Geometry: final body of the model. Coordinates: model frame, mm. Coordinates: 2 decimals unless noted, no trailing zeros. Loops run counter-clockwise (first coordinate to the right, second up) from the corner with the lowest first, then second, coordinate; pieces in that order, holes last. Notation, with made-up numbers: (32.25, -4) - (60.25, -4) arc R33 ccw to (60.25, 29) - close; hole circle Ø9 at (36, -10). An arc over 180 degrees is marked (long way). Put each result on its own line as item: value. Start each with the question number.
1) Section B-B on x = -31.55. Output: boundary loops of the cut face in (y, z), and give its area (3 significant figures).
2) Draft query along Y for faces 1 (the cylindrical face through (23.78, -24.3, 0.99)), 2 (the cylindrical face through (-0.1, 29.05, 0.99)), 3 (the cylindrical face through (24.3, 23.78, 0.99)). Return one class per face: +Y half, -Y half, draft (parallel to the pull), parting line (faces both ways), or undercut.
3) Material intervals for line 1 along Y through (x, z) = (0, 1.4); line 2 along X through (y, z) = (-1.5, 1.65); line 3 along Y through (x, z) = (-2, 0.7), sorted ascending. Write a range as from..to.
4) Section C-C on z = 1.6. Output: boundary loops of the cut face in (x, y).
5) Section A-A on y = 7.5. Output: boundary loops of the cut face in (x, z), and give its area (3 significant figures).
6) Section D-D on x = 24. Output: boundary loops of the cut face in (y, z).
7) Contact query for flat-ended pins moving along their axis: pin 1 Ø1 at (y, z) = (8, 1) entering from -X; pin 2 Ø5 at (x, y) = (-10, 11.5) entering from +Z. Output: stop coordinate, or through.
```python
from build123d import *

# Parameters (mm, degrees)
CYLINDER_R     = 2.5
CYLINDER_DEPTH = 10
ARRAY_COUNT    = 4
TUBE_R         = 34
TUBE_R_2       = 20
TUBE_DEPTH     = 2


with BuildPart() as array:
    # Cylinder → Cylinder (new body)
    with BuildSketch(Plane(origin=(31.55, 0, 0), x_dir=(1, 0, 0), z_dir=(0, 0, 1))):
        Circle(CYLINDER_R)
    extrude(amount=CYLINDER_DEPTH)

    # Array: Array ×4 about axis
    array_axis = Axis((0, 0, 0), (0, 0, 1))


with BuildPart() as array_1:
    add(array.part)
    for i in range(1, ARRAY_COUNT):
        add(array.part.rotate(array_axis, i * 360 / ARRAY_COUNT))


with BuildPart() as cut:
    # Tube → Tube (new body)
    with BuildSketch(Plane.XY):
        Circle(TUBE_R)
        Circle(TUBE_R_2, mode=Mode.SUBTRACT)
    extrude(amount=TUBE_DEPTH)

    # Cut: cut Array
    add(array_1.part, mode=Mode.SUBTRACT)


solid = cut.part
```
Answer block:
1. outline: (-12.67, 0) - (-2.5, 0) - (-2.5, 2) - (-12.67, 2) - close; (2.5, 0) - (12.67, 0) - (12.67, 2) - (2.5, 2) - close
1. area: 40.7 mm²
2. face 1: -Y half
2. face 2: undercut
2. face 3: +Y half
3. line 1: y = -29.05..-20, 20..29.05
3. line 2: x = -33.97..-33.55, -29.55..-19.94, 19.94..29.55, 33.55..33.97
3. line 3: y = -33.94..-33.05, -30.05..-19.9, 19.9..30.05, 33.05..33.94
4. outline: (-34, -0.52) arc R34 ccw to (-0.52, -34) arc R2.5 cw (long way) to (0.52, -34) arc R34 ccw to (34, -0.52) arc R2.5 cw (long way) to (34, 0.52) arc R34 ccw to (0.52, 34) arc R2.5 cw (long way) to (-0.52, 34) arc R34 ccw to (-34, 0.52) arc R2.5 cw (long way) to start; hole circle Ø40 at (0, 0)
5. outline: (-33.16, 0) - (-18.54, 0) - (-18.54, 2) - (-33.16, 2) - close; (18.54, 0) - (33.16, 0) - (33.16, 2) - (18.54, 2) - close
5. area: 58.5 mm²
6. outline: (-24.08, 0) - (24.08, 0) - (24.08, 2) - (-24.08, 2) - close
7. pin 1: stops at x = -33.16
7. pin 2: passes through
